Autodesk Inventor part; units mm, degrees
ref_plane "YZ Plane" through (0, 0, 0) normal (1, 0, 0) x (0, 1, 0)
ref_plane "XZ Plane" through (0, 0, 0) normal (0, 1, 0) x (-1, 0, 0)
ref_plane "XY Plane" through (0, 0, 0) normal (0, 0, 1) x (1, 0, 0)
sketch "Sketch1" plane through (0, 0, 0) normal (0, 1, 0) x (-1, 0, 0)
  line L0 (-304.8, 25.4) -> (-279.4, 25.4) construction
  line L1 (0, 25.4) -> (-25.4, 25.4) construction
  line L2 (0, 279.4) -> (-25.4, 279.4) construction
  line L3 (-304.8, 279.4) -> (-279.4, 279.4) construction
  circle A0 centre (-25.4, 279.4) radius 2.54
  circle A1 centre (-279.4, 279.4) radius 2.54
  circle A2 centre (-25.4, 25.4) radius 2.54
  circle A3 centre (-279.4, 25.4) radius 2.54
  line L4 (-304.8, 38.1) -> (-254, 38.1) construction
  circle A4 centre (-254, 38.1) radius 2.54
  line L5 (-304.8, 152.4) -> (-230.2081, 152.4) construction
  line L6 (-254, 38.1) -> (-209.55, 38.1) construction
  line L7 (-209.55, 38.1) -> (-146.05, 38.1) construction
  line L8 (-146.05, 38.1) -> (-17.526, 38.1) construction
  circle A5 centre (-209.55, 38.1) radius 2.54
  circle A6 centre (-146.05, 38.1) radius 2.54
  circle A7 centre (-17.526, 38.1) radius 2.54
  circle A8 centre (-254, 266.7) radius 2.54
  circle A9 centre (-209.55, 266.7) radius 2.54
  circle A10 centre (-146.05, 266.7) radius 2.54
  circle A11 centre (-17.526, 266.7) radius 2.54
  line L9 (-6.35, 298.45) -> (-298.45, 298.45)
  line L10 (-6.35, 6.35) -> (-298.45, 6.35)
  line L11 (0, 292.1) -> (0, 12.7)
  line L12 (-304.8, 12.7) -> (-304.8, 292.1)
  line L13 (-304.8, 152.4) -> (-292.1, 152.4)
  line L14 (-292.1, 152.4) -> (-292.1, 196.85)
  line L15 (-285.75, 203.2) -> (-273.05, 203.2)
  line L16 (-266.7, 196.85) -> (-266.7, 107.95)
  line L17 (-273.05, 101.6) -> (-285.75, 101.6)
  line L18 (-292.1, 107.95) -> (-292.1, 152.4)
  arc A12 (-285.75, 203.2) -> (-292.1, 196.85) centre (-285.75, 196.85) ccw
  arc A13 (-292.1, 107.95) -> (-285.75, 101.6) centre (-285.75, 107.95) ccw
  arc A14 (-273.05, 101.6) -> (-266.7, 107.95) centre (-273.05, 107.95) ccw
  arc A15 (-266.7, 196.85) -> (-273.05, 203.2) centre (-273.05, 196.85) ccw
  arc A16 (-304.8, 12.7) -> (-298.45, 6.35) centre (-298.45, 12.7) ccw
  arc A17 (-298.45, 298.45) -> (-304.8, 292.1) centre (-298.45, 292.1) ccw
  arc A18 (0, 292.1) -> (-6.35, 298.45) centre (-6.35, 292.1) ccw
  arc A19 (-6.35, 6.35) -> (0, 12.7) centre (-6.35, 12.7) ccw
  line L19 (-279.4, 25.4) -> (-241.3, 25.4) construction
  circle A20 centre (-241.3, 25.4) radius 2.54
  circle A21 centre (-241.3, 279.4) radius 2.54
  point P0 (0, 0)
  point P1 (-292.1, 203.2)
  point P2 (-266.7, 203.2)
  point P3 (-266.7, 101.6)
  point P4 (-292.1, 101.6)
  dimension "d3" = 25.4
  dimension "d5" = 25.4
  dimension "d7" = 25.4
  dimension "d9" = 25.4
  dimension "d10" = 5.08
  dimension "d11" = 5.08
  dimension "d12" = 5.08
  dimension "d13" = 5.08
  dimension "d15" = 50.8
  dimension "d16" = 5.08
  dimension "d18" = 44.45
  dimension "d19" = 63.5
  dimension "d20" = 128.524
  dimension "d21" = 5.08
  dimension "d22" = 5.08
  dimension "d23" = 5.08
  dimension "d27" = 50.8
  dimension "d28" = 25.4
  dimension "d29" = 101.6
  dimension "d31" = 6.35
  dimension "d32" = 6.35
  dimension "d33" = 6.35
  dimension "d34" = 6.35
  dimension "d35" = 6.35
  dimension "d38" = 38.1
  dimension "d39" = 5.08
extrude "Extrusion2" add sketch "Sketch1" along normal blind 6.35
properties part number "vrRig_v08_breadboardToSlideMount"
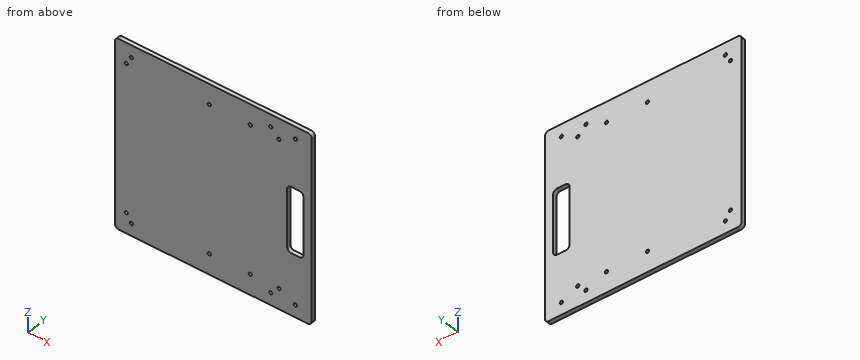
For this review, take the finished solid that the model builds, in its own axes (mm). Round coordinates to 2 decimals unless told otherwise and drop trailing zeros. Write each loop counter-clockwise with the first axis right and the second up, starting at its lowest first coordinate (ties: lowest second). Pieces come first, ordered by that corner, then holes. Notation, with made-up numbers: (8, 77.25) -> (20, 77.25) arc R16 ccw to (20, 84.25) -> close; hole circle Ø11 at (9, 29.5). An arc over 180 degrees is marked (long way). Use CSV: the item, a comma, the result in double quotes.
(1) To check wall thickness, follow L1, parallel to Z at x = 241.3, y = 2.25; L2, parallel to X at y = 2, z = 267; L3, parallel to X at y = 2.25, z = 107. State the ranges of each line that lie inside material, in increasing order. Write a range as [from, to].
Computed values:
L1,"[6.35, 22.86], [27.94, 276.86], [281.94, 298.45]"
L2,"[0, 15], [20.05, 143.53], [148.57, 207.03], [212.07, 251.48], [256.52, 304.8]"
L3,"[0, 266.77], [292.03, 304.8]"
(2) Clearance check with a flat-ended pin moving along its axis: P1, Ø4.5, axis at x = 25.4, z = 279.4, coming from the -Y side. State where the tip first meets the part, or that it passes through.
Computed values:
P1,"through"
(3) Consider section B-B, the plane y = 2.5. Give the number of separate pieces and of enclosed holes in the cut face, plus the area to 3 significant figures.
Computed values:
separate pieces,"1"
enclosed holes,"15"
area,"86,200 mm²"
(4) Consider section A-A, the plane z = 191. Give the boundary of the cut face in (x, y).
Computed values:
outline,"(0, 0) -> (266.7, 0) -> (266.7, 6.35) -> (0, 6.35) -> close; (292.1, 0) -> (304.8, 0) -> (304.8, 6.35) -> (292.1, 6.35) -> close"
